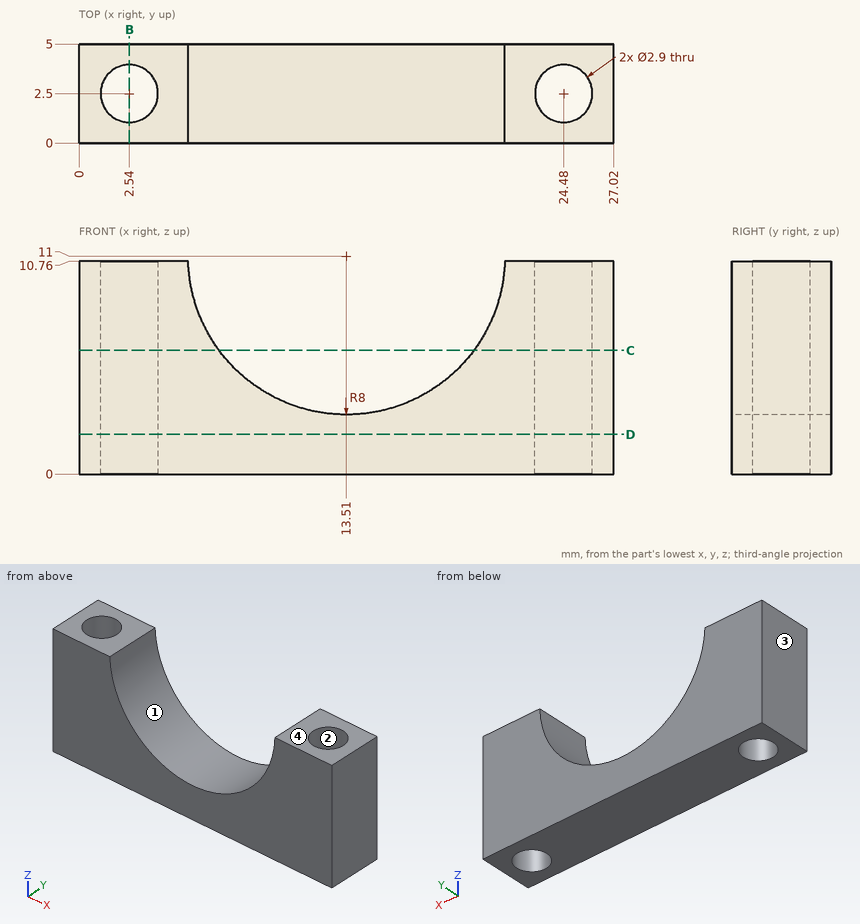
Geometry: see drawing. Coordinates: mm, zero at the bounding-box minimum. Round coordinates to 2 decimals unless told otherwise and drop trailing zeros. Loops run counter-clockwise (first coordinate to the right, second up) from the corner with the lowest first, then second, coordinate; pieces in that order, holes last.
(1) Contact query for flat-ended pins moving along their axis: pin 1 Ø3 at (x, y) = (10.5, 4.5) entering from +Z; pin 2 Ø2.5 at (x, y) = (2.54, 2.5) entering from +Z. Output: stop coordinate, or through.
From the geometry:
pin 1: stops at z = 4.39
pin 2: passes through
(2) Pull-direction query (X, two-part tool) for the marked faces 1, 2, 3 and 4; classes: +X half, -X half, draft (parallel to the pull), parting line (faces both ways), or undercut.
From the geometry:
face 1: undercut
face 2: undercut
face 3: -X half
face 4: draft
(3) Section query B-B (x = 2.54). Output: boundary loops of the cut face in (y, z).
From the geometry:
outline: (0, 0) - (1.05, 0) - (1.05, 10.76) - (0, 10.76) - close; (3.95, 0) - (5, 0) - (5, 10.76) - (3.95, 10.76) - close
(4) Material intervals for probe 1 along X at (y, z) = (2.5, 2.5); probe 2 along Y at (x, z) = (24.48, 6.25); probe 3 along X at (y, z) = (1.45, 8), sorted ascending.
From the geometry:
probe 1: x = 0 to 1.09, 3.99 to 23.03, 25.93 to 27.02
probe 2: y = 0 to 1.05, 3.95 to 5
probe 3: x = 0 to 1.54, 3.54 to 6.09, 20.93 to 23.48, 25.48 to 27.02
(5) Section query D-D (z = 2). Output: boundary loops of the cut face in (x, y).
From the geometry:
outline: (0, 0) - (27.02, 0) - (27.02, 5) - (0, 5) - close; hole circle Ø2.9 at (2.54, 2.5); hole circle Ø2.9 at (24.48, 2.5)
(6) Section query C-C (z = 6.25). Output: boundary loops of the cut face in (x, y), and give its area (3 significant figures).
From the geometry:
outline: (0, 0) - (7.07, 0) - (7.07, 5) - (0, 5) - close; (19.95, 0) - (27.02, 0) - (27.02, 5) - (19.95, 5) - close; hole circle Ø2.9 at (2.54, 2.5); hole circle Ø2.9 at (24.48, 2.5)
area: 57.5 mm2
